The listing builds one solid part. Answer for the finished solid, in the listing's coordinates (mm). Face numbers are marked on the shaded views. A direction names the side the tool comes from. Round coordinates to 2 decimals unless told otherwise and drop trailing zeros. Write each loop counter-clockwise with the first axis right and the second up, starting at its lowest first coordinate (ties: lowest second). Pieces come first, ordered by that corner, then holes. Notation, with made-up numbers: (-18, 74) -> (31, 74) arc R21 ccw to (31, 83) -> close; hole circle Ø4 at (20.25, 27.5). An arc over 180 degrees is marked (long way). Write each question's results on one line, items separated by ' | '. Start each with the question number.
```python
from build123d import *

# Parameters (mm, degrees)
F0_W      = 45
F0_H      = 100
F1_DEPTH  = 10.2
F2_W      = 17
F2_H      = 85
F3_DEPTH  = 8.6
F4_W      = 41.8
F4_H      = 100
F5_DEPTH  = 7
F8_R      = 8.5
F9_DEPTH  = 10
F14_W     = 131.8
F14_H     = 10.2
F15_DEPTH = 0.8


with BuildPart() as f1:
    # F0 (on Top) → F1 (new body)
    with BuildSketch(Plane.XY):
        with Locations((-33.8353561237, -14.8088461805)):
            Rectangle(F0_W, F0_H)
    extrude(amount=F1_DEPTH)

    # F2 (on face) → F3 (cut)
    with BuildSketch(Plane.XY.offset(10.2)):
        with Locations((-33.8353561237, -22.3088461805)):
            Rectangle(F2_W, F2_H)
    extrude(amount=-F3_DEPTH, mode=Mode.SUBTRACT)


with BuildPart() as f5:
    # F4 (on Top) → F5 (new body)
    with BuildSketch(Plane.XY):
        with Locations((-35.4353561237, -14.8088461805)):
            Rectangle(F4_W, F4_H)
    extrude(amount=F5_DEPTH)


with BuildPart() as f5_1:
    # F6: moved
    add(f5.part.moved(Location((1.6, 0, 1.6))))


with BuildPart() as f1_1:
    add(f1.part)

    # F7: cut F5
    add(f5_1.part, mode=Mode.SUBTRACT)


with BuildPart() as f9:
    # F8 (on Top) → F9 (new body)
    with BuildSketch(Plane.XY):
        with Locations((-33.8353561237, -64.8088461805)):
            Circle(F8_R)
    extrude(amount=F9_DEPTH)


with BuildPart() as f9_1:
    # F10: moved
    add(f9.part.moved(Location((0, 85, 4))))


with BuildPart() as f1_2:
    add(f1_1.part)

    # F11: cut F9
    add(f9_1.part, mode=Mode.SUBTRACT)


with BuildPart() as f12_1:
    # F12: copy of F1
    add(f1_2.part.moved(Location((43.4, 0, 0))))


with BuildPart() as f13_1:
    # F13: copy of F12_1
    add(f12_1.part.moved(Location((43.4, 0, 0))))


with BuildPart() as f1_3:
    add(f1_2.part)

    add(f12_1.part)  # F15 merges F12_1

    add(f13_1.part)  # F15 merges F13_1
    # F14 (on face) → F15 (join)
    with BuildSketch(Plane(origin=(0, 35.1911538195, 0), x_dir=(-1, 0, 0), z_dir=(0, 1, 0))):
        with Locations((-9.5646438763, 5.1)):
            Rectangle(F14_W, F14_H)
    extrude(amount=-F15_DEPTH)


solid = f1_3.part
```
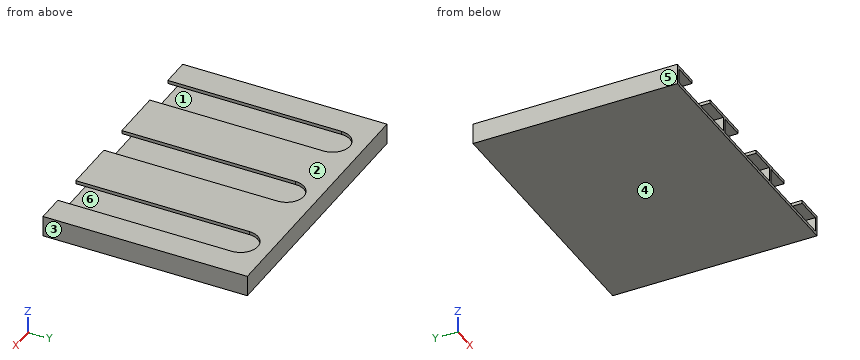
Q1. Each of these flat-tipped pins is pushed along its axis until it touches: pin 1 (5.5 mm diameter, centred on x = 62.5, z = 5.5, fed in from -Y); pin 2 (5 mm diameter, centred on x = -36, y = 10.5, fed in from +Z). Where does it stop, or does it pass through?
Q2. The part is cut by section C-C, the plane x = -8. Write down the section's boundary in (y, z).
Q3. The part is cut by section B-B, the plane y = -11.5. Write down the section's boundary in (x, z).
Q4. Determine the mould class of the marked faces 1, 2, 3 and 4 for opening direction Z: pulls with the +Z half, pulls with the -Z half, needs draft (parallel to the pull), parting line crosses it, or undercut.
Q5. The part is cut by section D-D, the plane x = 53. Write down the section's boundary in (y, z), then the cut area to 3 significant figures.
Q6. For the marked faces 5 and 6, determine the directions among +Z, -Z, +X, -X, +Y, -Y from which every point of the face is accessible in a straight line to the end or side of a thin tool.
Q7. The part is cut by section A-A, the plane z = 4.75. Write down the section's boundary in (x, y).
Q8. Find the intervals of material crossed by line 1 (X direction, y = -1.5, z = 9); line 2 (X direction, y = -49, z = 5); line 3 (Z direction, x = 20, y = -3), in increasing order.
Answers follow:
1) pin 1: y = 34.39 | pin 2: z = 1.6
2) outline: (-64.81, 0) -> (35.19, 0) -> (35.19, 10.2) -> (-64.81, 10.2) -> (-64.81, 8.6) -> (34.39, 8.6) -> (34.39, 1.6) -> (-64.81, 1.6) -> close
3) outline: (-56.34, 0) -> (75.46, 0) -> (75.46, 10.2) -> (61.46, 10.2) -> (61.46, 8.6) -> (73.86, 8.6) -> (73.86, 1.6) -> (32.06, 1.6) -> (32.06, 8.6) -> (44.46, 8.6) -> (44.46, 10.2) -> (18.06, 10.2) -> (18.06, 8.6) -> (30.46, 8.6) -> (30.46, 1.6) -> (-11.34, 1.6) -> (-11.34, 8.6) -> (1.06, 8.6) -> (1.06, 10.2) -> (-25.34, 10.2) -> (-25.34, 8.6) -> (-12.94, 8.6) -> (-12.94, 1.6) -> (-54.74, 1.6) -> (-54.74, 8.6) -> (-42.34, 8.6) -> (-42.34, 10.2) -> (-56.34, 10.2) -> close
4) face 1: undercut | face 2: pulls with the +Z half | face 3: needs draft | face 4: pulls with the -Z half
5) outline: (-64.81, 0) -> (35.19, 0) -> (35.19, 10.2) -> (28.69, 10.2) -> (28.69, 8.6) -> (34.39, 8.6) -> (34.39, 1.6) -> (-64.81, 1.6) -> close | area: 176 mm^2
6) face 5: +Z, -Z, -X, +Y, -Y | face 6: -Y
7) outline: (-56.34, -64.81) -> (-54.74, -64.81) -> (-54.74, 34.39) -> (-12.94, 34.39) -> (-12.94, -64.81) -> (-11.34, -64.81) -> (-11.34, 34.39) -> (30.46, 34.39) -> (30.46, -64.81) -> (32.06, -64.81) -> (32.06, 34.39) -> (73.86, 34.39) -> (73.86, -64.81) -> (75.46, -64.81) -> (75.46, 35.19) -> (-56.34, 35.19) -> close
8) line 1: -56.34 to -42.34, -25.34 to 1.06, 18.06 to 44.46, 61.46 to 75.46 | line 2: -56.34 to -54.74, -12.94 to -11.34, 30.46 to 32.06, 73.86 to 75.46 | line 3: 0 to 1.6, 8.6 to 10.2
